Model file for the job. Use its own axes, mm. Face numbers are marked on the shaded views. Give positions to 0.01 mm unless a question says otherwise; leave off trailing zeros. Loops run counter-clockwise (first coordinate to the right, second up) from the corner with the lowest first, then second, coordinate; pieces in that order, holes last. Notation, with made-up numbers: M 17,-5.75 L 69,-5.75 A31 cw 69,21.25 Z; hole C 10,76 d10. An arc over 180 degrees is marked long. Use CSV: the item, a comma, the result in double quotes. Start each with the question number.
(1) Wall check: line 1 along Y through (x, z) = (205.5, 81); line 2 along Y through (x, z) = (135.5, 79); line 3 along Y through (x, z) = (192, 47). Give the ranges that are in metal, low to high. Write a range as from..to.
(2) Two-plate mould, pull along Y, no slides. Class the marked faces 1 and 2: pulls with the +Y half, pulls with the -Y half, needs draft (parallel to the pull), parting line crosses it, or undercut.
(3) Slice it at A-A on y = 581. List the corners of the cut face in (x, z), and give its area (3 significant figures).
(4) Slice it at D-D on y = 285.5. List the corners of the cut face in (x, z).
(5) Slice it at B-B on x = 221. List the corners of the cut face in (y, z).
(6) Flat gauge pins, fed straight in: P1, Ø6, axis at y = 514.5, z = 61, coming from the -X side; P2, Ø5, axis at x = 229, z = 68.5, coming from the +Y side; P3, Ø22, axis at x = 192, z = 57.5, coming from the +Y side; P4, Ø5.5, axis at x = 227.32, y = 710.59, coming from the -Z side. Where does each tip first touch, or does it go through?
(7) Slice it at C-C on z = 79.5. State how many separate pieces and enclosed holes the cut face has, and give its area (3 significant figures).
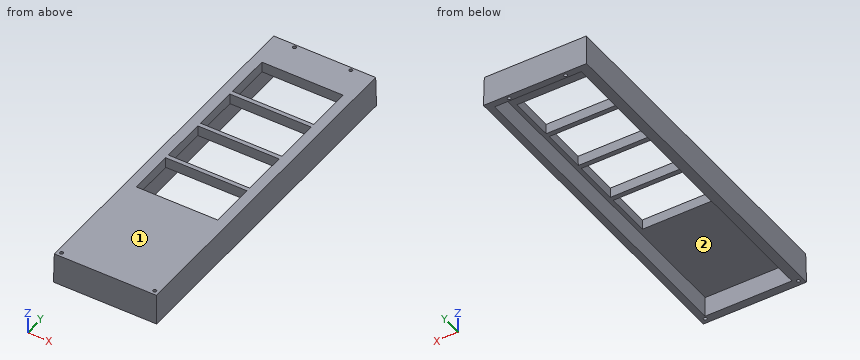
Autodesk Fusion 360 part; units mm, degrees
sketch "Sketch1" plane through (0, 0, 0) normal (0, 0, 1) x (1, 0, 0)
  line L0 (-23.9272, 0) -> (276.0728, 0)
  line L1 (276.0728, 0) -> (276.0728, 1000)
  line L2 (276.0728, 1000) -> (-23.9272, 1000)
  line L3 (-23.9272, 1000) -> (-23.9272, 0)
  line L4 (9.5728, 896.1324) -> (242.5728, 896.1324)
  line L5 (242.5728, 896.1324) -> (242.5728, 766.1324)
  line L6 (242.5728, 766.1324) -> (9.5728, 766.1324)
  line L7 (9.5728, 766.1324) -> (9.5728, 896.1324)
  line L8 (9.5728, 750.4224) -> (242.5728, 750.4224)
  line L9 (242.5728, 750.4224) -> (242.5728, 620.4224)
  line L10 (242.5728, 620.4224) -> (9.5728, 620.4224)
  line L11 (9.5728, 620.4224) -> (9.5728, 750.4224)
  line L12 (9.5728, 604.7124) -> (242.5728, 604.7124)
  line L13 (242.5728, 604.7124) -> (242.5728, 474.7124)
  line L14 (242.5728, 474.7124) -> (9.5728, 474.7124)
  line L15 (9.5728, 474.7124) -> (9.5728, 604.7124)
  line L16 (9.5728, 459.0024) -> (242.5728, 459.0024)
  line L17 (242.5728, 459.0024) -> (242.5728, 329.0024)
  line L18 (242.5728, 329.0024) -> (9.5728, 329.0024)
  line L19 (9.5728, 329.0024) -> (9.5728, 459.0024)
  dimension "d1" = 300
  dimension "d2" = 1000
  dimension "d3" = 130
  dimension "d4" = 130
  dimension "d5" = 233
  dimension "d6" = 233
  dimension "d7" = 33.5
  dimension "d8" = 33.5
  dimension "d9" = 15.71
  dimension "d10" = 15.71
  dimension "d11" = 15.71
  dimension "d12" = 15.71
  dimension "d13" = 15.71
  dimension "d14" = 15.71
extrude "Extrude1" add sketch "Sketch1" along normal blind 100 draft -1
sketch "Sketch2" plane through (0, 0, 0) normal (0, 0, 1) x (1, 0, 0)
  line L0 (256.197, 980.5748) -> (3.983, 980.5748)
  line L1 (3.983, 980.5748) -> (3.983, 23.2664)
  line L2 (3.983, 23.2664) -> (256.197, 23.2664)
  line L3 (256.197, 23.2664) -> (256.197, 980.5748)
extrude "Extrude2" cut sketch "Sketch2" along normal blind 70
hole "Hole1" at (-9.3135, 14.624, 100) direction (0, 0, -1) diameter 10 depth 100 tip angle 118
sketch "Sketch3" plane through (0, 0, 100) normal (0, 0, 1) x (-1, 0, 0)
  circle A0 centre (9.3135, -14.624) radius 5
  line L0 (-7.8273, -764.3868) -> (-7.8273, -897.8779)
  line L1 (-7.8273, -897.8779) -> (-244.3183, -897.8779)
  line L2 (-244.3183, -897.8779) -> (-244.3183, -764.3868)
  line L3 (-244.3183, -764.3868) -> (-7.8273, -764.3868)
  line L4 (-7.8273, -618.6768) -> (-7.8273, -752.1679)
  line L5 (-7.8273, -752.1679) -> (-244.3183, -752.1679)
  line L6 (-244.3183, -752.1679) -> (-244.3183, -618.6768)
  line L7 (-244.3183, -618.6768) -> (-7.8273, -618.6768)
  line L8 (-7.8273, -472.9668) -> (-7.8273, -606.4579)
  line L9 (-7.8273, -606.4579) -> (-244.3183, -606.4579)
  line L10 (-244.3183, -606.4579) -> (-244.3183, -472.9668)
  line L11 (-244.3183, -472.9668) -> (-7.8273, -472.9668)
  line L12 (-7.8273, -327.2568) -> (-7.8273, -460.7479)
  line L13 (-7.8273, -460.7479) -> (-244.3183, -460.7479)
  line L14 (-244.3183, -460.7479) -> (-244.3183, -327.2568)
  line L15 (-244.3183, -327.2568) -> (-7.8273, -327.2568)
  line L16 (-274.3273, -998.2545) -> (22.1817, -998.2545)
  line L17 (22.1817, -998.2545) -> (22.1817, -1.7455)
  line L18 (22.1817, -1.7455) -> (-274.3273, -1.7455)
  line L19 (-274.3273, -1.7455) -> (-274.3273, -998.2545)
  circle A1 centre (-261.4591, -14.624) radius 5
  point P0 (-126.0728, -1.7455)
  dimension "d22" = 12.8682
  dimension "d23" = 12.8785
hole "Hole2" at (261.4591, 14.624, 100) direction (0, 0, -1) diameter 10 depth 119 tip angle 118
hole "Hole3" at (207.9885, 988.9182, 100) direction (0, 0, -1) diameter 10 depth 120 tip angle 118
sketch "Sketch4" plane through (0, 0, 100) normal (0, 0, 1) x (-1, 0, 0)
  circle A0 centre (-207.9885, -988.9182) radius 5
  circle A1 centre (-261.4591, -14.624) radius 5
  circle A2 centre (9.3135, -14.624) radius 5
  line L0 (-7.8273, -764.3868) -> (-7.8273, -897.8779)
  line L1 (-7.8273, -897.8779) -> (-244.3183, -897.8779)
  line L2 (-244.3183, -897.8779) -> (-244.3183, -764.3868)
  line L3 (-244.3183, -764.3868) -> (-7.8273, -764.3868)
  line L4 (-7.8273, -618.6768) -> (-7.8273, -752.1679)
  line L5 (-7.8273, -752.1679) -> (-244.3183, -752.1679)
  line L6 (-244.3183, -752.1679) -> (-244.3183, -618.6768)
  line L7 (-244.3183, -618.6768) -> (-7.8273, -618.6768)
  line L8 (-7.8273, -472.9668) -> (-7.8273, -606.4579)
  line L9 (-7.8273, -606.4579) -> (-244.3183, -606.4579)
  line L10 (-244.3183, -606.4579) -> (-244.3183, -472.9668)
  line L11 (-244.3183, -472.9668) -> (-7.8273, -472.9668)
  line L12 (-7.8273, -327.2568) -> (-7.8273, -460.7479)
  line L13 (-7.8273, -460.7479) -> (-244.3183, -460.7479)
  line L14 (-244.3183, -460.7479) -> (-244.3183, -327.2568)
  line L15 (-244.3183, -327.2568) -> (-7.8273, -327.2568)
  line L16 (-274.3273, -998.2545) -> (22.1817, -998.2545)
  line L17 (22.1817, -998.2545) -> (22.1817, -1.7455)
  line L18 (22.1817, -1.7455) -> (-274.3273, -1.7455)
  line L19 (-274.3273, -1.7455) -> (-274.3273, -998.2545)
  circle A3 centre (-44.157, -988.9182) radius 5
  point P0 (-126.0728, -998.2545)
  dimension "d39" = 163.8315
extrude "Extrude3" cut sketch "Sketch4" against normal blind 300 contours A3
sketch "Sketch5" plane through (0, 765.899, 13.3688) normal (0, 0.9998, 0.0175) x (-1, 0, 0)
  line L0 (-243.7946, 56.6398) -> (-8.3509, 56.6398)
  line L1 (-8.3509, 56.6398) -> (-7.8273, 86.6444)
  line L2 (-7.8273, 86.6444) -> (-244.3183, 86.6444)
  line L3 (-244.3183, 86.6444) -> (-243.7946, 56.6398)
  dimension "d32" = 30.0046
sketch "Sketch6" plane through (-23.9199, 0, 0.4175) normal (-0.9998, 0, 0.0175) x (0, -1, 0)
  line L0 (-1.7455, 99.5976) -> (-998.2545, 99.5976)
  line L1 (-998.2545, 99.5976) -> (-1000, -0.4176)
  line L2 (-1000, -0.4176) -> (0, -0.4176)
  line L3 (0, -0.4176) -> (-1.7455, 99.5976)
  dimension "d33" = 100.0152
scale "Scale1" factor 0.46 about (243.7946, 473.4905, 70) bodies 1
sketch "Sketch7" plane through (0, 0, 83.8) normal (0, 0, 1) x (-1, 0, 0)
  line L0 (-257.8396, -714.8819) -> (-121.4455, -714.8819)
  line L1 (-121.4455, -714.8819) -> (-121.4455, -256.4878)
  line L2 (-121.4455, -256.4878) -> (-257.8396, -256.4878)
  line L3 (-257.8396, -256.4878) -> (-257.8396, -714.8819)
  line L4 (-135.2496, -406.223) -> (-135.2496, -467.6289)
  line L5 (-135.2496, -467.6289) -> (-244.0355, -467.6289)
  line L6 (-244.0355, -467.6289) -> (-244.0355, -406.223)
  line L7 (-244.0355, -406.223) -> (-135.2496, -406.223)
  line L8 (-135.2496, -473.2496) -> (-135.2496, -534.6555)
  line L9 (-135.2496, -534.6555) -> (-244.0355, -534.6555)
  line L10 (-244.0355, -534.6555) -> (-244.0355, -473.2496)
  line L11 (-244.0355, -473.2496) -> (-135.2496, -473.2496)
  line L12 (-135.2496, -540.2762) -> (-135.2496, -601.6821)
  line L13 (-135.2496, -601.6821) -> (-244.0355, -601.6821)
  line L14 (-244.0355, -601.6821) -> (-244.0355, -540.2762)
  line L15 (-244.0355, -540.2762) -> (-135.2496, -540.2762)
  line L16 (-135.2496, -607.3028) -> (-135.2496, -668.7087)
  line L17 (-135.2496, -668.7087) -> (-244.0355, -668.7087)
  line L18 (-244.0355, -668.7087) -> (-244.0355, -607.3028)
  line L19 (-244.0355, -607.3028) -> (-135.2496, -607.3028)
  circle A0 centre (-127.3649, -262.4119) radius 2.3
  circle A1 centre (-251.9203, -262.4119) radius 2.3
  circle A2 centre (-227.3238, -710.5872) radius 2.3
  circle A3 centre (-151.9613, -710.5872) radius 2.3
  dimension "d35" = 61.4059
  dimension "d36" = 108.7859
sketch "Sketch8" plane through (0, 716.1265, 12.5) normal (0, 0.9998, 0.0175) x (-1, 0, 0)
  line L0 (-121.4455, 71.3108) -> (-257.8396, 71.3108)
  line L1 (-257.8396, 71.3108) -> (-258.6426, 25.3038)
  line L2 (-258.6426, 25.3038) -> (-120.6426, 25.3038)
  line L3 (-120.6426, 25.3038) -> (-121.4455, 71.3108)
  line L4 (-257.8396, 71.3108) -> (-121.4455, 71.3108)
  dimension "d37" = 46.007
sketch "Sketch9" plane through (0, 0, 83.8) normal (0, 0, 1) x (-1, 0, 0)
  circle A0 centre (-151.9613, -710.5872) radius 2.3
  point P0 (-185, -715)
  point P1 (-187.4151, -715)
  point P2 (-227.3238, -710.5872)
  point P3 (-151.9613, -710.5872)
  dimension "d38" = 4.6
  dimension "d40" = 75.3625
sketch "Sketch10" plane through (0, 0, 83.8) normal (0, 0, 1) x (-1, 0, 0)
  line L0 (-257.8396, -256.4878) -> (-257.8396, -714.8819)
  line L1 (-121.4455, -714.8819) -> (-121.4455, -256.4878)
  line L2 (-121.4455, -256.4878) -> (-257.8396, -256.4878)
  circle A0 centre (-151.9613, -710.5872) radius 2.3
  line L3 (-257.8396, -714.8819) -> (-121.4455, -714.8819)
  point P0 (-127.3649, -262.4119)
  point P1 (-151.9613, -710.5872)
  dimension "d41" = 136.3941
  dimension "d42" = 458.3941
  dimension "d43" = 5.9194
  dimension "d44" = 5.9241
  dimension "d45" = 4.6
  dimension "d46" = 4.2947
  dimension "d47" = 30.5158
extrude "Extrude4" cut 1 faces at (126.6208, 562.1575, 37.8) along direction (0, 0, 1) blind 5
Reply:
1,line 1,"y = 256.44..406.27, 467.58..473.3, 534.61..540.33, 601.63..607.35, 668.66..714.93"
1,line 2,"y = 256.4..406.31, 467.55..473.33, 534.57..540.36, 601.6..607.39, 668.62..714.97"
1,line 3,"y = 255.85..266.39, 706.75..715.52"
2,face 1,"needs draft"
2,face 2,"undercut"
3,outline,"M 120.73,42.8 L 133.48,42.8 L 133.48,70 L 135.49,70 L 135.25,83.8 L 121.45,83.8 Z; M 243.79,70 L 249.5,70 L 249.5,42.8 L 258.56,42.8 L 257.84,83.8 L 244.04,83.8 Z"
3,area,"968 mm^2"
4,outline,"M 120.73,42.8 L 133.48,42.8 L 133.48,70 L 249.5,70 L 249.5,42.8 L 258.56,42.8 L 257.84,83.8 L 121.45,83.8 Z"
5,outline,"M 255.77,42.8 L 266.39,42.8 L 266.39,70 L 406.46,70 L 406.22,83.8 L 256.49,83.8 Z; M 467.39,70 L 473.49,70 L 473.25,83.8 L 467.63,83.8 Z; M 534.41,70 L 540.52,70 L 540.28,83.8 L 534.66,83.8 Z; M 601.44,70 L 607.54,70 L 607.3,83.8 L 601.68,83.8 Z; M 668.47,70 L 706.75,70 L 706.75,42.8 L 715.6,42.8 L 714.88,83.8 L 668.71,83.8 Z"
6,P1,"stops at x = 121"
6,P2,"stops at y = 715.19"
6,P3,"stops at y = 715.53"
6,P4,"stops at z = 42.8"
7,separate pieces,"1"
7,enclosed holes,"8"
7,area,"35,900 mm^2"
